The model under review builds one solid part; all positions refer to its coordinate system, in mm. Face numbers are marked on the shaded views. Coordinates: 2 decimals unless noted, no trailing zeros. Loops run counter-clockwise (first coordinate to the right, second up) from the corner with the lowest first, then second, coordinate; pieces in that order, holes last. Notation, with made-up numbers: (73.25, -29.75) - (100.25, -29.75) arc R36 cw to (100.25, 6.25) - close; hole circle Ø7 at (-37, 30.25). An arc over 180 degrees is marked (long way). Use a Markdown table: item, result. Add a question column.
1) Clearance check with a flat-ended pin moving along its axis: pin 1 (6 mm diameter, centred on x = 7.29, z = 12.45, fed in from -Y) (3 decimals). State where the tip first meets the part, or that it passes through.
2) The part is to be moulded in two halves that separate along X. For the marked faces 1, 2, 3 and 4, say which applies: pulls with the +X half, pulls with the -X half, needs draft (parallel to the pull), parting line crosses it, or undercut.
3) To check wall thickness, follow L1, parallel to Z at x = 58, y = -4.5; L2, parallel to X at y = -4.75, z = 18.75; L3, parallel to X at y = -1.25, z = 12.5. State the ranges of each line that lie inside material, in increasing order. Write a range as [from, to].
4) Add section D-D, the plane z = 13.75. Give the boundary of the cut face in (x, y) (3 decimals).
5) Add section B-B, the plane z = 17.75. Give the boundary of the cut face in (x, y) (3 decimals), and give its area (3 significant figures).
6) Add section A-A, the plane y = -5.25. Give the boundary of the cut face in (x, z), and give its area (3 significant figures).
```python
from build123d import *

# Parameters (mm, degrees)
F0_W     = 63.5
F0_H     = 25.4
F0_W_2   = 56.649408
F0_H_2   = 15.184378
F1_DEPTH = 6.35
F2_DEPTH = 3.175
F3_R     = 2.54
F4_DEPTH = 25.4


with BuildPart() as f1:
    # F0 (on Front) → F1 (new body)
    with BuildSketch(Plane.XZ):
        with Locations((31.75, 12.7)):
            Rectangle(F0_W, F0_H)
        with Locations((31.390783, 12.702317)):
            Rectangle(F0_W_2, F0_H_2, mode=Mode.SUBTRACT)
    extrude(amount=F1_DEPTH)

    # F0 (on Front) → F2 (join)
    with BuildSketch(Plane.XZ):
        with Locations((31.390783, 12.702317)):
            Rectangle(F0_W_2, F0_H_2)
    extrude(amount=F2_DEPTH)

    # F3 (on Front) → F4 (cut)
    with BuildSketch(Plane.XZ):
        with Locations((7.289108, 12.447039)):
            Circle(F3_R)
    extrude(amount=F4_DEPTH, mode=Mode.SUBTRACT)


solid = f1.part
```
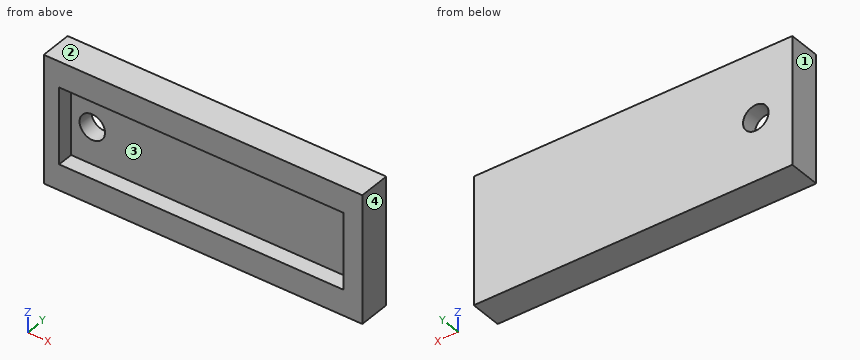
From the geometry:
| question | item | result |
|---|---|---|
| 1 | pin 1 | stops at y = -3.175 |
| 2 | face 1 | pulls with the -X half |
| 2 | face 2 | needs draft |
| 2 | face 3 | undercut |
| 2 | face 4 | pulls with the +X half |
| 3 | L1 | z = [0, 5.11], [20.29, 25.4] |
| 3 | L2 | x = [0, 3.07], [59.72, 63.5] |
| 3 | L3 | x = [0, 4.75], [9.83, 63.5] |
| 4 | outline | (0, -6.35) - (3.066, -6.35) - (3.066, -3.175) - (5.109, -3.175) - (5.109, 0) - (0, 0) - close; (9.469, -3.175) - (59.715, -3.175) - (59.715, -6.35) - (63.5, -6.35) - (63.5, 0) - (9.469, 0) - close |
| 5 | outline | (0, -6.35) - (3.066, -6.35) - (3.066, -3.175) - (59.715, -3.175) - (59.715, -6.35) - (63.5, -6.35) - (63.5, 0) - (0, 0) - close |
| 5 | area | 223 mm^2 |
| 6 | outline | (0, 0) - (63.5, 0) - (63.5, 25.4) - (0, 25.4) - close; hole (3.07, 5.11) - (59.72, 5.11) - (59.72, 20.29) - (3.07, 20.29) - close |
| 6 | area | 753 mm^2 |
